from build123d import *

# Parameters (mm, degrees)
SKETCH_1_W          = 6.4
SKETCH_1_H          = 12
EXTRUDE_1_DEPTH     = 5
SKETCH_2_R          = 2.5
EXTRUDE_2_DEPTH     = 2
SKETCH_3_R          = 0.8
EXTRUDE_3_DEPTH     = 0.5
SKETCH_4_W          = 1
SKETCH_4_H          = 0.25
EXTRUDE_4_DEPTH     = 1
SKETCH_5_R          = 1.8
CUT_EXTRUDE_1_DEPTH = 16.447977214
SKETCH_6_W          = 1
SKETCH_6_H          = 0.25
EXTRUDE_5_DEPTH     = 1


with BuildPart() as part:
    # 草图1 → 凸台-拉伸1 (new body)
    with BuildSketch(Plane(origin=(0, 0, 0), x_dir=(1, 0, 0), z_dir=(0, 1, 0))):
        with Locations((0, 6)):
            Rectangle(SKETCH_1_W, SKETCH_1_H)
    extrude(amount=EXTRUDE_1_DEPTH)

    # 草图2 → 凸台-拉伸2 (add)
    with BuildSketch(Plane.XY):
        with Locations(Location((0, 2.5, 0), (0, 0, 270))):
            Circle(SKETCH_2_R)
    extrude(amount=EXTRUDE_2_DEPTH)

    # 草图3 → 凸台-拉伸3 (add)
    with BuildSketch(Plane.XZ):
        with Locations(Location((0, -3, 0), (0, 0, 270))):
            Circle(SKETCH_3_R)
        with Locations(Location((0, -9, 0), (0, 0, 270))):
            Circle(SKETCH_3_R)
    extrude(amount=EXTRUDE_3_DEPTH)

    # 草图4 → 凸台-拉伸4 (add)
    with BuildSketch(Plane(origin=(3.2, 0, 0), x_dir=(0, 0, -1), z_dir=(1, 0, 0))):
        with Locations((1.95, 0.125)):
            Rectangle(SKETCH_4_W, SKETCH_4_H)
        with Locations((5.25, 0.125)):
            Rectangle(SKETCH_4_W, SKETCH_4_H)
        with Locations((9.75, 0.125)):
            Rectangle(SKETCH_4_W, SKETCH_4_H)
    extrude(amount=EXTRUDE_4_DEPTH)

    # 草图5 → 切除-拉伸1 (cut, through all)
    with BuildSketch(Plane.XY.offset(2)):
        with Locations((0, 2.5)):
            Circle(SKETCH_5_R)
    extrude(amount=-CUT_EXTRUDE_1_DEPTH, mode=Mode.SUBTRACT)

    # 草图6 → 凸台-拉伸5 (add)
    with BuildSketch(Plane.ZY.offset(3.2)):
        with Locations((-2.5, 0.125)):
            Rectangle(SKETCH_6_W, SKETCH_6_H)
        with Locations((-7.5, 0.125)):
            Rectangle(SKETCH_6_W, SKETCH_6_H)
    extrude(amount=EXTRUDE_5_DEPTH)


solid = part.part
Geometry: final body of the model. Coordinates: model frame, mm. A direction names the side the tool comes from. Round coordinates to 2 decimals unless told otherwise and drop trailing zeros. Loops run counter-clockwise (first coordinate to the right, second up) from the corner with the lowest first, then second, coordinate; pieces in that order, holes last.
Q1. Section C-C on x = 0.5. Return loops of the section in (y, z), plus the area to 3 significant figures.
Q2. Material intervals for L1, parallel to Y at x = 0, z = -3.25; L2, parallel to Y at x = 0, z = -1.25; L3, parallel to X at y = 2.85, z = -7.5, sorted ascending.
Q3. Pull-direction query (X, two-part tool) for faces 1 (the cylindrical face through (-0.234, 4.285, -4.902)), 2 (the cylindrical face through (0.24, -0.246, -3.763)), 3 (the flat face through (-3.7, 0.25, -2.5)); classes: released by +X, released by -X, zero draft, split by the parting line, or undercut.
Q4. Pin query (flat end, axial travel): P1, Ø1.5, axis at y = 2.5, z = -5, coming from the +X side; P2, Ø2.5, axis at x = -1, z = -4.5, coming from the -Y side; P3, Ø3, axis at x = 0, y = 2.5, coming from the +Z side; P4, Ø1.5, axis at x = 2, z = -3, coming from the -Y side. Return the tip coordinate at first contact, or that it passes through.
Q5. Section B-B on y = 3.9. Return loops of the section in (x, z).
Q6. Section A-A on z = -9. Return loops of the section in (x, y), plus the area to 3 significant figures.
Q7. Access query for faces 4 (the cylindrical face through (0.54, -0.25, -8.41)), 5 (the flat face through (-3, 2, 0)), 6 (the flat face through (4, 0.25, -10)). Directions: +Z, -Z, +X, -X, +Y, -Y. A direction counts if a zero-diameter tool reaches every point of the face in a straight line with its end or side. Return the directions, or none.
Q8. Section D-D on y = 2.5. Return loops of the section in (x, z), plus the area to 3 significant figures.
Evaluation:
1. outline: (-0.5, -9.62) - (0, -9.62) - (0, -12) - (0.77, -12) - (0.77, 2) - (0.05, 2) - (0.05, 0) - (0, 0) - (0, -2.38) - (-0.5, -2.38) - (-0.5, -3.62) - (0, -3.62) - (0, -8.38) - (-0.5, -8.38) - close; (4.23, -12) - (5, -12) - (5, 0) - (4.95, 0) - (4.95, 2) - (4.23, 2) - close
1. area: 22.6 mm2
2. L1: y = -0.5 to 0.7, 4.3 to 5
2. L2: y = 0 to 0.7, 4.3 to 5
2. L3: x = -3.2 to -1.77, 1.77 to 3.2
3. face 1: undercut
3. face 2: split by the parting line
3. face 3: zero draft
4. P1: stops at x = 3.2
4. P2: stops at y = -0.5
4. P3: passes through
4. P4: stops at y = 0
5. outline: (-3.2, -12) - (-1.13, -12) - (-1.13, 2) - (-2.07, 2) - (-2.07, 0) - (-3.2, 0) - close; (1.13, -12) - (3.2, -12) - (3.2, 0) - (2.07, 0) - (2.07, 2) - (1.13, 2) - close
6. outline: (-3.2, 0) - (-0.8, 0) - (-0.8, -0.5) - (0.8, -0.5) - (0.8, 0) - (3.2, 0) - (3.2, 5) - (-3.2, 5) - close; hole circle Ø3.6 at (0, 2.5)
6. area: 22.6 mm2
7. face 4: -Y
7. face 5: +Z, -X
7. face 6: +Z, -Z, +X, +Y
8. outline: (-3.2, -12) - (-1.8, -12) - (-1.8, 2) - (-2.5, 2) - (-2.5, 0) - (-3.2, 0) - close; (1.8, -12) - (3.2, -12) - (3.2, 0) - (2.5, 0) - (2.5, 2) - (1.8, 2) - close
8. area: 36.4 mm2
